```python
from build123d import *

# Parameters (mm, degrees)
SKETCH1_W           = 50
SKETCH1_H           = 40
BOSS_EXTRUDE2_DEPTH = 5
SKETCH2_W           = 2
SKETCH2_H           = 40
BOSS_EXTRUDE4_DEPTH = 12
SKETCH3_W           = 10
SKETCH3_H           = 40
BOSS_EXTRUDE5_DEPTH = 5
SKETCH5_R           = 1.5
BOSS_EXTRUDE6_DEPTH = 7
FILLET1_R           = 10
BOSS_EXTRUDE7_START = -7
SKETCH6_R           = 1.5
BOSS_EXTRUDE7_DEPTH = 7
FILLET2_R           = 10


with BuildPart() as part:
    # Sketch1 → Boss-Extrude2 (new body)
    with BuildSketch(Plane(origin=(0, 0, 0), x_dir=(1, 0, 0), z_dir=(0, 1, 0))):
        with Locations((25, 20)):
            Rectangle(SKETCH1_W, SKETCH1_H)
    extrude(amount=BOSS_EXTRUDE2_DEPTH)

    # Sketch2 → Boss-Extrude4 (add)
    with BuildSketch(Plane(origin=(0, 5, 0), x_dir=(1, 0, 0), z_dir=(0, 1, 0))):
        with Locations((1, 20)):
            Rectangle(SKETCH2_W, SKETCH2_H)
        with Locations((49, 20)):
            Rectangle(SKETCH2_W, SKETCH2_H)
    extrude(amount=BOSS_EXTRUDE4_DEPTH)

    # Sketch3 → Boss-Extrude5 (add)
    with BuildSketch(Plane(origin=(0, 17, 0), x_dir=(1, 0, 0), z_dir=(0, 1, 0))):
        with Locations((5, 20)):
            Rectangle(SKETCH3_W, SKETCH3_H)
        with Locations((45, 20)):
            Rectangle(SKETCH3_W, SKETCH3_H)
    extrude(amount=BOSS_EXTRUDE5_DEPTH)

    # Sketch5 → Boss-Extrude6 (add)
    with BuildSketch(Plane.ZY):
        with BuildLine():
            Line((-40, 22), (-35, 22))
            Line((-35, 22), (-35, 26))
            ThreePointArc((-35, 26), (-37.5, 28.5), (-40, 26))
            Line((-40, 26), (-40, 22))
        make_face()
        with Locations((-37.5, 24.41459259)):
            Circle(SKETCH5_R, mode=Mode.SUBTRACT)
    extrude(amount=-BOSS_EXTRUDE6_DEPTH)

    # Fillet1
    # the kernel refuses this fillet: 10 mm, written as the material it adds along each edge
    with BuildSketch(Plane(origin=(0, 22, -35), x_dir=(0, 0.99826370600864, -0.058903083670516616), z_dir=(1, 0, 0))) as fillet1_piece_1:
        with BuildLine():
            CenterArc((9.48397203, 9.040187721), FILLET1_R, 183.376852724, 61.314597986)
            Line((-0.49866503, 8.451156885), (-1.496928736, 8.392253801))
            Line((-1.496928736, 8.392253801), (-0.998263706, -0.058903084))
            Line((-0.998263706, -0.058903084), (0.058903084, -0.998263706))
            ThreePointArc((0.058903084, -0.998263706), (4.051957908, -0.762651371), (4.781551673, -0.904018772))
            Line((4.781551673, -0.904018772), (5.209044433, 0))
        make_face()
    extrude(amount=7)

    # Sketch6 → Boss-Extrude7 (add)
    with BuildSketch(Plane(origin=(50, 0, 0), x_dir=(0, 0, -1), z_dir=(1, 0, 0)).offset(BOSS_EXTRUDE7_START)):
        with BuildLine():
            Line((35, 22), (40, 22))
            Line((40, 22), (40, 26))
            ThreePointArc((40, 26), (37.5, 28.5), (35, 26))
            Line((35, 26), (35, 22))
        make_face()
        with Locations(Location((37.5, 24.41459259, 0), (0, 0, 180))):
            Circle(SKETCH6_R, mode=Mode.SUBTRACT)
    extrude(amount=BOSS_EXTRUDE7_DEPTH)

    # Fillet2
    # the kernel refuses this fillet: 10 mm, written as the material it adds along each edge
    with BuildSketch(Plane(origin=(43, 22, -35), x_dir=(0, 0, 1), z_dir=(1, 0, 0))) as fillet2_piece_1:
        with BuildLine():
            CenterArc((8.4658561, -10), FILLET2_R, 90, 61.314597986)
            Line((-0.30682878, -5.2), (-1.184097268, -4.72))
            ThreePointArc((-1.184097268, -4.72), (-1, -4), (-1, 0))
            Line((-1, 0), (0, 1))
            Line((0, 1), (8.4658561, 1))
            Line((8.4658561, 1), (8.4658561, 0))
        make_face()
    extrude(amount=7)


solid = part.part
```
Geometry check sheet. Reference: the model listing, model coordinates, mm. A direction names the side the tool comes from. Coordinates: 2 decimals unless noted, no trailing zeros. Write each loop counter-clockwise with the first axis right and the second up, starting at its lowest first coordinate (ties: lowest second). Pieces come first, ordered by that corner, then holes. Notation, with made-up numbers: M -36.5,28.5 L -2.5,28.5 A10 cw -2.5,37.5 Z; hole C 43.5,85 d2. An arc over 180 degrees is marked long. Answer as a JSON object with one key per item and string values.
1. Section check A-A, the plane z = -37.5. Enter the section's corners in (x, y), plus the area to 3 significant figures.
Answers below:
{"outline": "M 0,0 L 50,0 L 50,22.91 L 43,22.91 L 43,22 L 40,22 L 40,17 L 48,17 L 48,5 L 2,5 L 2,17 L 10,17 L 10,22 L 7,22 L 7,22.91 L 0,22.91 Z; M 0,25.91 L 7,25.91 L 7,28.5 L 0,28.5 Z; M 43,25.91 L 50,25.91 L 50,28.5 L 43,28.5 Z", "area": "447 mm²"}
2. Draft check along Y on faces 1 (the cylindrical face through (46.45, 25.33, -38.69)), 2 (the flat face through (23, 4, -40)), 3 (the flat face through (25, 5, -20)), 4 (the cylindrical face through (46.45, 23.36, -31.57)). Enter one of: released by +Y, released by -Y, zero draft, split by the parting line, or undercut.
Answers below:
{"face 1": "undercut", "face 2": "zero draft", "face 3": "undercut", "face 4": "released by +Y"}
3. Go/stop test with flat-tipped pins: pin 1 Ø5 at (x, z) = (43.5, -14) entering from +Y; pin 2 Ø8 at (x, z) = (4, -26) entering from +Y; pin 3 Ø12 at (x, z) = (30.5, -20) entering from +Y. Record where each tip stops, or that it passes through.
Answers below:
{"pin 1": "stops at y = 22", "pin 2": "stops at y = 22.62", "pin 3": "stops at y = 5"}
4. Section check D-D, the plane z = -22.5. Enter the section's corners in (x, y).
Answers below:
{"outline": "M 0,0 L 50,0 L 50,22 L 40,22 L 40,17 L 48,17 L 48,5 L 2,5 L 2,17 L 10,17 L 10,22 L 0,22 Z"}
5. Tool access check on faces 5 (the flat face through (6, 17, -20)), 6 (the flat face through (10, 19, -20)), 7 (the flat face through (0, 11, -20)). Record the directions out of +Z, -Z, +X, -X, +Y, -Y that give a thin tool (end or side, any length) a straight path to the whole face; none if there is none.
Answers below:
{"face 5": "+Z, -Z", "face 6": "+Z, -Z, +Y", "face 7": "+Z, -Z, -X, +Y, -Y"}
6. Section check C-C, the plane y = 9.25. Enter the section's corners in (x, z).
Answers below:
{"outline": "M 0,-40 L 2,-40 L 2,0 L 0,0 Z; M 48,-40 L 50,-40 L 50,0 L 48,0 Z"}
7. Section check B-B, the plane y = 20.25. Enter the section's corners in (x, z), plus the area to 3 significant figures.
Answers below:
{"outline": "M 0,-40 L 10,-40 L 10,0 L 0,0 Z; M 40,-40 L 50,-40 L 50,0 L 40,0 Z", "area": "800 mm²"}
8. Scan lines: L1, parallel to Y at x = 5, z = -37.5; L2, parallel to X at y = 9.5, z = -19; L3, parallel to Y at x = 45, z = -7. Record each from-to range of solid material in increasing order.
Answers below:
{"L1": "y = 0 to 5, 17 to 22.91, 25.91 to 28.5", "L2": "x = 0 to 2, 48 to 50", "L3": "y = 0 to 5, 17 to 22"}
